Autodesk Inventor part; units mm, degrees
ref_plane "YZ Plane" through (0, 0, 0) normal (1, 0, 0) x (0, 1, 0)
ref_plane "XZ Plane" through (0, 0, 0) normal (0, 1, 0) x (-1, 0, 0)
ref_plane "XY Plane" through (0, 0, 0) normal (0, 0, 1) x (1, 0, 0)
sketch "Sketch1" plane through (0, 0, 0) normal (0, 1, 0) x (-1, 0, 0)
  line L0 (0, 0) -> (-203.2, 0)
  line L1 (-203.2, 0) -> (-203.2, -184.15)
  line L2 (-203.2, -184.15) -> (0, -184.15)
  line L3 (0, -184.15) -> (0, 0)
  dimension "blength" = 203.2
  dimension "bwidth" = 184.15
extrude "Extrusion1" add sketch "Sketch1" along normal blind 152.4
shell "Shell1" thickness 6.35 removed faces 2 at (135.4667, 50.8, -184.15) at (67.7333, 50.8, 0)
fillet "Fillet1" radius 1.27 24 edges at (0, 152.4, -92.075) (101.6, 152.4, -184.15) (203.2, 152.4, -92.075) (101.6, 152.4, 0) (0, 76.2, -184.15) (6.35, 76.2, -184.15) (196.85, 76.2, -184.15) (101.6, 6.35, -184.15) (101.6, 146.05, -184.15) (203.2, 76.2, -184.15) (101.6, 0, -184.15) (6.35, 6.35, -92.075) (6.35, 146.05, -92.075) (196.85, 6.35, -92.075) (196.85, 146.05, -92.075) (6.35, 76.2, 0) (101.6, 6.35, 0) (196.85, 76.2, 0) (101.6, 146.05, 0) (0, 76.2, 0) (0, 0, -92.075) (101.6, 0, 0) (203.2, 76.2, 0) (203.2, 0, -92.075)
sketch "Sketch9" plane through (203.2, 1.27, -182.88) normal (1, 0, 0) x (0, 0, -1)
  line L0 (0, 0) -> (-181.61, 0)
  line L1 (0, 149.86) -> (0, 0)
  line L2 (-181.61, 0) -> (-181.61, 149.86)
  circle A0 centre (-135.5725, 76.2) radius 6.35
  circle A1 centre (-46.0375, 76.2) radius 6.35
  point P0 (-182.88, -1.27)
  dimension "csize" = 12.7
  dimension "d81" = 12.7
  dimension "d82" = 76.2
  dimension "d83" = 76.2
  dimension "d84" = 46.0375
  dimension "d85" = 46.0375
extrude "Extrusion6" cut sketch "Sketch9" against normal blind 6.35
sketch "Sketch10" plane through (0, 1.27, -1.27) normal (-1, 0, 0) x (0, 0, 1)
  line L0 (0, 0) -> (-181.61, 0)
  line L1 (0, 149.86) -> (0, 0)
  line L2 (-181.61, 0) -> (-181.61, 149.86)
  line L3 (0, 0) -> (-181.61, 0)
  line L4 (0, 149.86) -> (0, 0)
  line L5 (-181.61, 0) -> (-181.61, 149.86)
  circle A0 centre (-135.5725, 76.2) radius 6.35
  circle A1 centre (-46.0375, 76.2) radius 6.35
  point P0 (1.27, -1.27)
  point P1 (-182.88, -1.27)
  dimension "d106" = 12.7
  dimension "d107" = 12.7
  dimension "d108" = 46.0375
  dimension "d109" = 46.0375
  dimension "d110" = 76.2
  dimension "d111" = 76.2
sketch "Sketch11" plane through (0, 152.4, 0) normal (0, 1, 0) x (1, 0, 0)
  line L0 (201.93, 1.27) -> (1.27, 1.27)
  line L1 (201.93, 182.88) -> (201.93, 1.27)
  line L2 (1.27, 182.88) -> (201.93, 182.88)
  circle A0 centre (38.1, 136.8425) radius 6.35
  circle A1 centre (101.6, 136.8425) radius 6.35
  circle A2 centre (165.1, 136.8425) radius 6.35
  circle A3 centre (44.45, 47.3075) radius 6.35
  circle A4 centre (107.95, 47.3075) radius 6.35
  circle A5 centre (161.29, 47.3075) radius 6.35
  line L3 (1.27, 1.27) -> (1.27, 182.88)
  point P0 (0, 0)
  dimension "d112" = 12.7
  dimension "d113" = 12.7
  dimension "d114" = 12.7
  dimension "d115" = 46.0375
  dimension "d116" = 46.0375
  dimension "d117" = 46.0375
  dimension "d118" = 12.7
  dimension "d119" = 12.7
  dimension "d120" = 12.7
  dimension "d126" = 46.0375
  dimension "d127" = 46.0375
  dimension "d128" = 46.0375
  dimension "d134" = 40.64
  dimension "d135" = 106.68
extrude "Extrusion7" cut sketch "Sketch11" against normal blind 6.35 contours A0 | A1 | A2 | A3 | A4 | A5
extrude "Extrusion8" cut sketch "Sketch10" against normal blind 6.35
equation "\"d81\" = csize"
equation "\"d82\" = 0.5 * bheight"
equation "\"d83\" = 0.5 * bheight"
equation "\"d84\" = 0.25 * bwidth"
equation "\"d85\" = 0.25 * bwidth"
equation "\"d106\" = csize"
equation "\"d107\" = csize"
equation "\"d108\" = 0.25 * bwidth"
equation "\"d109\" = 0.25 * bwidth"
equation "\"d110\" = 0.5 * bheight"
equation "\"d111\" = 0.5 * bheight"
equation "\"d112\" = csize"
equation "\"d113\" = csize"
equation "\"d114\" = csize"
equation "\"d115\" = 0.25 * bwidth"
equation "\"d116\" = 0.25 * bwidth"
equation "\"d117\" = 0.25 * bwidth"
equation "\"d118\" = csize"
equation "\"d119\" = csize"
equation "\"d120\" = csize"
equation "\"d126\" = 0.25 * bwidth"
equation "\"d127\" = 0.25 * bwidth"
equation "\"d128\" = 0.25 * bwidth"
equation "\"d130\" = holeextrude"
equation "\"d132\" = holeextrude"
equation "\"topCircDistFromCntr\" = 0.2 * bwidth"
properties part number "Box Base"
Build history of the part. All positions in model axes, mm. A direction names the side the tool comes from. Round coordinates to 2 decimals unless told otherwise and drop trailing zeros. Write each loop counter-clockwise with the first axis right and the second up, starting at its lowest first coordinate (ties: lowest second). Pieces come first, ordered by that corner, then holes.
1) Pin check, flat tip, straight feed: pin 1 (7.5 mm diameter, centred on x = 44.45, z = -47.31, fed in from +Y). Stop position of the tip, or through.
2) Drill centre lines: probe 1 along Z at (x, y) = (202, 77); probe 2 along Y at (x, z) = (160, -64); probe 3 along X at (y, z) = (116, -150). Where is each one in solid material? Low to high.
3) Band-saw the part on D-D, the plane y = 96. List the corners of the cut face in (x, z), and give its area (3 significant figures).
4) Band-saw the part on C-C, the plane z = -32.5. List the corners of the cut face in (x, y).
5) Mould opens along Z. For faces 1 (the cylindrical face through (3.13, 82.82, -43.89)), 2 (the flat face through (103, 152.4, -91)), 3 (the flat face through (4.5, 75.9, 0)), 4 (the flat face through (199, 76, -184.15)) say: +Z half, -Z half, draft (parallel to the pull), parting line (faces both ways), or undercut.
6) Band-saw the part on A-A, the plane y = 77.47. Give the number of separate pieces and of enclosed holes in the cut face, and give its area (3 significant figures).
7) Band-saw the part on B-B, the plane x = 179. List the corners of the cut face in (y, z), and give its area (3 significant figures).
8) 3-axis set-ups, long thin cutter, end or side, ignore diameter. For faces 5 (the flat face through (196.85, 75, -91)), 6 (the cylindrical face through (107.466, 149.269, -134.41)), 7 (the cylindrical face through (200.069, 81.762, -42.627)): which of +Z, -Z, +X, -X, +Y, -Y reach the whole face in a straight line?
Ans:
1. pin 1: stops at y = 6.35
2. probe 1: z = -184.15 to -143.18, -130.51 to -53.64, -40.97 to 0
2. probe 2: y = 0 to 6.35, 146.05 to 152.4
2. probe 3: x = 0 to 6.35, 196.85 to 203.2
3. outline: (0, -182.88) arc R1.27 ccw to (1.27, -184.15) - (5.08, -184.15) arc R1.27 ccw to (6.35, -182.88) - (6.35, -1.27) arc R1.27 ccw to (5.08, 0) - (1.27, 0) arc R1.27 ccw to (0, -1.27) - close; (196.85, -182.88) arc R1.27 ccw to (198.12, -184.15) - (201.93, -184.15) arc R1.27 ccw to (203.2, -182.88) - (203.2, -1.27) arc R1.27 ccw to (201.93, 0) - (198.12, 0) arc R1.27 ccw to (196.85, -1.27) - close
3. area: 2,340 mm2
4. outline: (0, 1.27) arc R1.27 ccw to (1.27, 0) - (201.93, 0) arc R1.27 ccw to (203.2, 1.27) - (203.2, 151.13) arc R1.27 ccw to (201.93, 152.4) - (1.27, 152.4) arc R1.27 ccw to (0, 151.13) - close; hole (6.35, 7.62) arc R1.27 ccw to (7.62, 6.35) - (195.58, 6.35) arc R1.27 ccw to (196.85, 7.62) - (196.85, 144.78) arc R1.27 ccw to (195.58, 146.05) - (7.62, 146.05) arc R1.27 ccw to (6.35, 144.78) - close
5. face 1: undercut
5. face 2: draft
5. face 3: +Z half
5. face 4: -Z half
6. separate pieces: 6
6. enclosed holes: 0
6. area: 2,010 mm2
7. outline: (0, -182.88) arc R1.27 ccw to (1.27, -184.15) - (5.08, -184.15) arc R1.27 ccw to (6.35, -182.88) - (6.35, -1.27) arc R1.27 ccw to (5.08, 0) - (1.27, 0) arc R1.27 ccw to (0, -1.27) - close; (146.05, -182.88) arc R1.27 ccw to (147.32, -184.15) - (151.13, -184.15) arc R1.27 ccw to (152.4, -182.88) - (152.4, -1.27) arc R1.27 ccw to (151.13, 0) - (147.32, 0) arc R1.27 ccw to (146.05, -1.27) - close
7. area: 2,340 mm2
8. face 5: +Z, -Z
8. face 6: +Y
8. face 7: +X, -X
